Read the model definition and answer for the solid it produces. Units are mm, in the model's axes. Face numbers are marked on the shaded views. A direction names the side the tool comes from. Coordinates: 2 decimals unless noted, no trailing zeros. Write each loop counter-clockwise with the first axis right and the second up, starting at its lowest first coordinate (ties: lowest second). Pieces come first, ordered by that corner, then holes.
Item 1: Section A-A (y = 0) is taken. Give the vertices of the cut face in (x, z), then the cut area to 3 significant figures.
Item 2: Section C-C (y = 6) is taken. Give the vertices of the cut face in (x, z).
Item 3: Straight lines are drawn through the part: probe 1 along Y at (x, z) = (70.5, 2); probe 2 along Y at (x, z) = (-21, 2.25); probe 3 along X at (y, z) = (5.5, 7). For each, find the intervals that lie inside material, in ascending order.
Item 4: Section B-B (z = 1.5) is taken. Give the vertices of the cut face in (x, y).
Item 5: A tool of negligible diameter and unlimited length cuts with its end or side. For the marked faces 1 and 2, from which of +Z, -Z, +X, -X, +Y, -Y can it reach the whole face along a straight path? Write none if from no direction.
Item 6: Determine the mould class of the marked faces 3, 4 and 5 for opening direction X: released by +X, released by -X, zero draft, split by the parting line, or undercut.
Item 7: Each of these flat-tipped pins is pushed along its axis until it touches: P1, Ø2, axis at x = 23.5, z = 8.5, coming from the -Y side; P2, Ø4, axis at x = 13, z = 7.5, coming from the +Y side; P3, Ø1.5, axis at x = 43, y = -6.5, coming from the -Z side. Where does it stop, or does it pass through?
Item 8: Section D-D (x = 15.5) is taken. Give the vertices of the cut face in (y, z), then the cut area to 3 significant figures.
from build123d import *

# Parameters (mm, degrees)
IZIM1_R                     = 10.5
Y_KSEKLIK_EKSTR_ZYON1_DEPTH = 10


with BuildPart() as part:
    # Çizim1 → Yükseklik-Ekstrüzyon1 (new body)
    with BuildSketch(Plane.XY):
        with BuildLine():
            Line((80.295084686, 5), (-11.098302389, 5))
            ThreePointArc((-11.098302389, 5), (-40.240438013, 0), (-11.098302389, -5))
            Line((-11.098302389, -5), (80.295084686, -5))
            Line((80.295084686, -5), (80.295084686, 5))
        make_face()
        with Locations((-25.240438013, 0)):
            Circle(IZIM1_R, mode=Mode.SUBTRACT)
    extrude(amount=Y_KSEKLIK_EKSTR_ZYON1_DEPTH)


solid = part.part
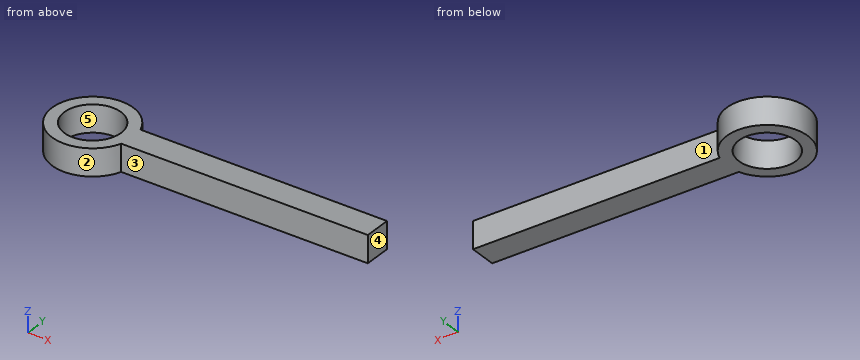
Established:
1. outline: (-40.24, 0) - (-35.74, 0) - (-35.74, 10) - (-40.24, 10) - close; (-14.74, 0) - (80.3, 0) - (80.3, 10) - (-14.74, 10) - close
1. area: 995 mm2
2. outline: (-38.99, 0) - (-33.86, 0) - (-33.86, 10) - (-38.99, 10) - close; (-16.62, 0) - (-11.49, 0) - (-11.49, 10) - (-16.62, 10) - close
3. probe 1: y = -5 to 5
3. probe 2: y = -14.39 to -9.61, 9.61 to 14.39
3. probe 3: x = -39.2 to -34.18, -16.3 to -11.29
4. outline: (-11.1, -5) - (80.3, -5) - (80.3, 5) - (-11.1, 5) arc R15 ccw (long way) to start; hole circle Ø21 at (-25.24, 0)
5. face 1: +Z, -Z, +X, +Y
5. face 2: +Z, -Z
6. face 3: zero draft
6. face 4: released by +X
6. face 5: undercut
7. P1: stops at y = -5
7. P2: stops at y = 5
7. P3: passes through
8. outline: (-5, 0) - (5, 0) - (5, 10) - (-5, 10) - close
8. area: 100 mm2
